Model file for the job. Use its own axes, mm. Coordinates: 2 decimals unless noted, no trailing zeros. Write each loop counter-clockwise with the first axis right and the second up, starting at its lowest first coordinate (ties: lowest second). Pieces come first, ordered by that corner, then holes.
Q1. Band-saw the part on A-A, the plane x = -438. Write the cut outline in (y, z), plus the area to 3 significant figures.
Q2. Pin check, flat tips, straight feed: P1, Ø2, axis at x = -735.5, y = 12.5, coming from the +Z side; P2, Ø7, axis at x = -396.5, y = 35, coming from the +Z side; P3, Ø4, axis at x = -867, y = 23.5, coming from the +Z side. Stop position of each tip, or through.
Q3. Band-saw the part on B-B, the plane z = 25. Write the cut outline in (x, y), plus the area to 3 significant figures.
Q4. Pull direction Z, two halves, no side cores. Call faces 1 (the cylindrical face through (-493, 20, 33)), 2 (the flat face through (-493, 20, 0)), 3 (the flat face through (0, 20, 13)): released by +Z, released by -Z, zero draft, split by the parting line, or undercut.
Q5. Drill centre lines: probe 1 along Y at (x, z) = (-950, 3.15); probe 2 along Z at (x, y) = (-220, 32); probe 3 along Y at (x, z) = (-283, 25). Where is each one in solid material? Low to high.
from build123d import *

# Parameters (mm, degrees)
F1_DEPTH = 1000
F2_R     = 2.5
F3_DEPTH = 33.001


with BuildPart() as f1:
    # F0 (on Right) → F1 (new body)
    with BuildSketch(Plane.YZ):
        with BuildLine():
            Line((0, 5), (0, 0))
            Line((0, 0), (40, 0))
            Line((40, 0), (40, 5))
            Line((40, 5), (31, 5))
            Line((31, 5), (31, 10))
            Line((31, 10), (27, 10))
            Line((27, 10), (23.471015, 17.792222))
            ThreePointArc((23.471015, 17.792222), (20, 33), (16.528985, 17.792222))
            Line((16.528985, 17.792222), (13, 10))
            Line((13, 10), (9, 10))
            Line((9, 10), (9, 5))
            Line((9, 5), (0, 5))
        make_face()
    extrude(amount=-F1_DEPTH)

    # F2 (on face) → F3 (cut, through all)
    with BuildSketch(Plane(origin=(0, 0, 0), x_dir=(1, 0, 0), z_dir=(0, 0, -1))):
        with Locations((-50, -5)):
            Circle(F2_R)
        with Locations((-200, -5)):
            Circle(F2_R)
        with Locations((-350, -5)):
            Circle(F2_R)
        with Locations((-500, -5)):
            Circle(F2_R)
        with Locations((-650, -5)):
            Circle(F2_R)
        with Locations((-800, -5)):
            Circle(F2_R)
        with Locations((-950, -5)):
            Circle(F2_R)
        with Locations((-950, -35)):
            Circle(F2_R)
        with Locations((-800, -35)):
            Circle(F2_R)
        with Locations((-650, -35)):
            Circle(F2_R)
        with Locations((-500, -35)):
            Circle(F2_R)
        with Locations((-350, -35)):
            Circle(F2_R)
        with Locations((-200, -35)):
            Circle(F2_R)
        with Locations((-50, -35)):
            Circle(F2_R)
    extrude(amount=-F3_DEPTH, mode=Mode.SUBTRACT)


solid = f1.part
Answer sheet:
1. outline: (0, 0) - (40, 0) - (40, 5) - (31, 5) - (31, 10) - (27, 10) - (23.47, 17.79) arc R8 ccw (long way) to (16.53, 17.79) - (13, 10) - (9, 10) - (9, 5) - (0, 5) - close
1. area: 589 mm2
2. P1: stops at z = 29.66
2. P2: stops at z = 5
2. P3: stops at z = 32.86
3. outline: (-1000, 12) - (0, 12) - (0, 28) - (-1000, 28) - close
3. area: 16,000 mm2
4. face 1: undercut
4. face 2: released by -Z
4. face 3: zero draft
5. probe 1: y = 0 to 2.5, 7.5 to 32.5, 37.5 to 40
5. probe 2: z = 0 to 5
5. probe 3: y = 12 to 28
